```python
from build123d import *

# Parameters (mm, degrees)
F1_W     = 50.793938
F1_H     = 50.793942
F2_DEPTH = 25.4
F3_DEPTH = 25.4


with BuildPart() as f2:
    # F1 (on Front) → F2 (new body)
    with BuildSketch(Plane.XZ):
        with Locations((-15.085418, 14.70351)):
            Rectangle(F1_W, F1_H)
    extrude(amount=-F2_DEPTH)

    # F0 (on Front) → F3 (join)
    with BuildSketch(Plane.XZ):
        Polygon((-15.276372, 40.100481), (-40.673342, 40.100481), (-40.673342, -10.693461), (10.120596, -10.693461), (10.120596, 14.703508), (-15.276372, 14.703508), align=None)
    extrude(amount=F3_DEPTH)


solid = f2.part
```
For this review, take the finished solid that the model builds, in its own axes (mm). A direction names the side the tool comes from. Round coordinates to 2 decimals unless told otherwise and drop trailing zeros. Order: outer loops, then holes, each group sorted by start corner. A loop starts at its lowest first (then second) coordinate and runs counter-clockwise, first axis right, second up.
Q1. Insertion check: P1, Ø20.5, axis at y = -15, z = 25.5, coming from the +X side; P2, Ø20.5, axis at y = 15.5, z = 12.5, coming from the -X side; P3, Ø6, axis at x = 0.5, z = 27, coming from the -Y side. Each pin has a flat end and moves straight along its axis. Give the tip position at first contact, or say it passes through.
Findings below:
P1: stops at x = -15.28
P2: stops at x = -40.48
P3: stops at y = 0
Q2. We need section A-A, the plane z = 28.5. Give the boundary of the cut face in (x, y), plus the area to 3 significant figures.
Findings below:
outline: (-40.67, -25.4) - (-15.28, -25.4) - (-15.28, 0) - (10.31, 0) - (10.31, 25.4) - (-40.48, 25.4) - (-40.48, 0) - (-40.67, 0) - close
area: 1,940 mm2
Q3. We need section B-B, the plane x = -7. Give the boundary of the cut face in (y, z).
Findings below:
outline: (-25.4, -10.69) - (25.4, -10.69) - (25.4, 40.1) - (0, 40.1) - (0, 14.7) - (-25.4, 14.7) - close
Q4. Machinability: for faces 1 (the flat face through (-40.673, -13, 15)), 2 (the flat face through (-40.482, 13, 14)), 3 (the flat face through (-20, 6, 40.1)), 4 (the flat face through (-15.276, -13, 27)), 5 (the flat face through (10.121, -13, 2)), which of the approach directions +Z, -Z, +X, -X, +Y, -Y give a long, thin tool a straight path to every point of the face, cutting with its end or side? Answer none if there is none.
Findings below:
face 1: +Z, -Z, -X, +Y, -Y
face 2: +Z, -Z, -X, +Y
face 3: +Z, +X, -X, +Y, -Y
face 4: +Z, +X, -Y
face 5: +Z, -Z, +X, -Y
Q5. We need section C-C, the plane y = -13.5. Give the boundary of the cut face in (x, z), plus the area to 3 significant figures.
Findings below:
outline: (-40.67, -10.69) - (10.12, -10.69) - (10.12, 14.7) - (-15.28, 14.7) - (-15.28, 40.1) - (-40.67, 40.1) - close
area: 1,940 mm2
Q6. Wall thickness on line 1 (X direction, y = -12, z = 29.5); line 2 (X direction, y = 11, z = 23.5); line 3 (Y direction, x = -11, z = 34): over which ranges is each line inside the solid? List them lowest first.
Findings below:
line 1: x = -40.67 to -15.28
line 2: x = -40.48 to 10.31
line 3: y = 0 to 25.4
